```python
from build123d import *

# Parameters (mm, degrees)
SKETCH1_W                  = 1498.6
SKETCH1_H                  = 596.9
BOSS_EXTRUDE1_DEPTH        = 25.4
SKETCH3_W                  = 38.1
SKETCH3_H                  = 38.1
BOSS_EXTRUDE2_DEPTH        = 917.575
SKETCH4_W                  = 508
SKETCH4_H                  = 38.1
BOSS_EXTRUDE3_DEPTH        = 38.1
F_1_2_0_5_DIAMETER_HOLE1_D = 12.7
SKETCH9_W                  = 1409.7
SKETCH9_H                  = 520.7
SKETCH9_W_2                = 1397
SKETCH9_H_2                = 508
BOSS_EXTRUDE4_DEPTH        = 76.2
F_1_1_DIAMETER_HOLE3_D     = 25.4


with BuildPart() as part:
    # Sketch1 → Boss-Extrude1 (new body)
    with BuildSketch(Plane(origin=(0, 0, 0), x_dir=(1, 0, 0), z_dir=(0, 1, 0))):
        Rectangle(SKETCH1_W, SKETCH1_H)
    extrude(amount=BOSS_EXTRUDE1_DEPTH)

    # Sketch3 → Boss-Extrude2 (add)
    with BuildSketch(Plane.XZ.offset(-25.4)):
        with Locations((-679.45, 234.95)):
            Rectangle(SKETCH3_W, SKETCH3_H)
        with Locations((679.45, 234.95)):
            Rectangle(SKETCH3_W, SKETCH3_H)
        with Locations((679.45, -234.95)):
            Rectangle(SKETCH3_W, SKETCH3_H)
        with Locations((-679.45, -234.95)):
            Rectangle(SKETCH3_W, SKETCH3_H)
    extrude(amount=BOSS_EXTRUDE2_DEPTH)

    # Sketch4 → Boss-Extrude3 (add)
    with BuildSketch(Plane(origin=(698.5, 0, 0), x_dir=(0, 0, -1), z_dir=(1, 0, 0))):
        with Locations((0, -323.85)):
            Rectangle(SKETCH4_W, SKETCH4_H)
    boss_extrude3 = extrude(amount=-BOSS_EXTRUDE3_DEPTH)

    # Mirror1: Boss-Extrude3 across plane
    add(boss_extrude3.mirror(Plane(origin=(0, 0, 0), x_dir=(0, 0, 1), z_dir=(1, 0, 0))))

    # 1/2 (0.5) Diameter Hole1 (through all)
    with Locations(Plane(origin=(0, 25.4, 0), x_dir=(1, 0, 0), z_dir=(0, 1, 0))):
        with Locations((277.712499946, 0)):
            Hole(F_1_2_0_5_DIAMETER_HOLE1_D / 2)

    # Sketch9 → Boss-Extrude4 (add)
    with BuildSketch(Plane.XZ):
        Rectangle(SKETCH9_W, SKETCH9_H)
        Rectangle(SKETCH9_W_2, SKETCH9_H_2, mode=Mode.SUBTRACT)
    extrude(amount=BOSS_EXTRUDE4_DEPTH)

    # 1 (1) Diameter Hole3 (through all)
    with Locations(Plane(origin=(0, 25.4, 0), x_dir=(1, 0, 0), z_dir=(0, 1, 0))):
        with Locations((277.712499946, -63.5)):
            Hole(F_1_1_DIAMETER_HOLE3_D / 2)


solid = part.part
```
Design review of the part built by this model. Coordinates are the model's own, in mm. A direction names the side the tool comes from. Coordinates: 2 decimals unless noted, no trailing zeros. Order: outer loops, then holes, each group sorted by start corner. A loop starts at its lowest first (then second) coordinate and runs counter-clockwise, first axis right, second up.
1) Take a section at B-B, the plane z = 182. Give the boundary of the cut face in (x, y).
2) Mouldability with a two-part tool opening along Y and no side actions: class faces 4 (the flat face through (-10, -38, 260.35)), 5 (the flat face through (-680, -150, 215.9)), 6 (the flat face through (679, -892.175, 235)) as +Y half, -Y half, draft (parallel to the pull), parting line (faces both ways), or undercut.
3) Take a section at C-C, the plane x = -143.5. Give the boundary of the cut face in (y, z), and give its area (3 significant figures).
4) Wall thickness on line 1 along X through (y, z) = (-367.5, -220.5); line 2 along Z through (x, y) = (205, -36.5); line 3 along Y through (x, z) = (301, 169): over which ranges is each line inside the solid? List them lowest first.
5) Clearance check with flat-ended pins moving along their axes: pin 1 (1 mm diameter, centred on x = -415, z = -237, fed in from -Y); pin 2 (19 mm diameter, centred on x = 686, y = -303.5, fed in from +Z); pin 3 (19 mm diameter, centred on x = 687, y = -663.5, fed in from -Z). State where each tip first meets the part, or that it passes through.
6) Take a section at A-A, the plane y = -697. Give the boundary of the cut face in (x, z).
7) For faces 1 (the flat face through (-9, -38, 254)), 2 (the flat face through (680, -342.9, 3)), 3 (the flat face through (679, -150, 215.9)), list the 3-axis set-ups (+Z, -Z, +X, -X, +Y, -Y) from which the entire face can be reached by the end or side of a thin tool; tool diameter is ignored.
Returned:
1. outline: (-749.3, 0) - (-704.85, 0) - (-704.85, -76.2) - (-698.5, -76.2) - (-698.5, 0) - (698.5, 0) - (698.5, -76.2) - (704.85, -76.2) - (704.85, 0) - (749.3, 0) - (749.3, 25.4) - (-749.3, 25.4) - close; (-698.5, -342.9) - (-660.4, -342.9) - (-660.4, -304.8) - (-698.5, -304.8) - close; (660.4, -342.9) - (698.5, -342.9) - (698.5, -304.8) - (660.4, -304.8) - close
2. face 4: draft
2. face 5: undercut
2. face 6: -Y half
3. outline: (-76.2, -260.35) - (0, -260.35) - (0, -298.45) - (25.4, -298.45) - (25.4, 298.45) - (0, 298.45) - (0, 260.35) - (-76.2, 260.35) - (-76.2, 254) - (0, 254) - (0, -254) - (-76.2, -254) - close
3. area: 16,100 mm2
4. line 1: x = -698.5 to -660.4, 660.4 to 698.5
4. line 2: z = -260.35 to -254, 254 to 260.35
4. line 3: y = 0 to 25.4
5. pin 1: stops at y = 0
5. pin 2: stops at z = 254
5. pin 3: stops at z = -254
6. outline: (-698.5, -254) - (-660.4, -254) - (-660.4, -215.9) - (-698.5, -215.9) - close; (-698.5, 215.9) - (-660.4, 215.9) - (-660.4, 254) - (-698.5, 254) - close; (660.4, -254) - (698.5, -254) - (698.5, -215.9) - (660.4, -215.9) - close; (660.4, 215.9) - (698.5, 215.9) - (698.5, 254) - (660.4, 254) - close
7. face 1: -Y
7. face 2: +X, -X, -Y
7. face 3: none
